For this review, take the finished solid that the model builds, in its own axes (mm). A direction names the side the tool comes from. Round coordinates to 2 decimals unless told otherwise and drop trailing zeros. Order: outer loops, then holes, each group sorted by start corner. A loop starts at its lowest first (then second) coordinate and runs counter-clockwise, first axis right, second up. Notation, with made-up numbers: (-33, -28.75) - (8, -28.75) arc R26 cw to (8, 4.25) - close; hole circle Ø2 at (50.25, 43). An arc over 180 degrees is marked (long way). One line per item, written item: value.
Autodesk Inventor part; units mm, degrees
ref_plane "YZ Plane" through (0, 0, 0) normal (1, 0, 0) x (0, 1, 0)
ref_plane "XZ Plane" through (0, 0, 0) normal (0, 1, 0) x (-1, 0, 0)
ref_plane "XY Plane" through (0, 0, 0) normal (0, 0, 1) x (1, 0, 0)
sketch "Esquisse3" plane through (0, 0, 0) normal (0, 1, 0) x (-1, 0, 0)
  line L0 (0, 0) -> (11.196, -1.161)
  line L1 (11.196, -1.161) -> (11.196, -3.161)
  line L2 (11.196, -3.161) -> (0, -2)
  line L3 (0, -2) -> (-8.226, -2.628)
  line L4 (-8.226, -2.628) -> (-8.226, -0.628)
  line L5 (-8.226, -0.628) -> (0, 0)
  line L6 (0, 0) -> (0, -2) construction
  dimension "d10" = 0.628
  dimension "d11" = 1.161
  dimension "d12" = 11.256
  dimension "d13" = 8.226
  dimension "d14" = 2
extrude "Extrusion1" add sketch "Esquisse3" along normal blind 8
ref_plane "Plan de construction1" through (0, 10, 0) normal (0, 1, 0) x (1, 0, 0)
sketch "Esquisse4" plane through (0, 10, 0) normal (0, 1, 0) x (1, 0, 0)
  line L0 (8.226, 0.628) -> (8.226, 2.628) construction
  line L1 (8.226, 2.628) -> (0, 2) construction
  line L2 (8.226, 2.628) -> (0, 2) construction
  line L3 (0, 2) -> (-11.196, 3.161) construction
  line L4 (0, 2) -> (-11.196, 3.161) construction
  line L5 (-11.196, 3.161) -> (-11.196, 4.661) construction
  line L6 (-11.196, 4.661) -> (0, 3.5)
  line L7 (0, 3.5) -> (8.226, 4.128)
  line L8 (8.226, 2.628) -> (8.226, 4.128) construction
  line L9 (0, 2) -> (0, 3.5) construction
  line L10 (-11.196, 4.661) -> (-11.196, 6.0463)
  line L11 (-11.196, 6.0463) -> (-0.0003, 4.8853)
  line L12 (-0.0003, 4.8853) -> (8.226, 5.5133)
  line L13 (8.226, 5.5133) -> (8.226, 4.128)
  point P0 (0, 0)
  dimension "d18" = 1.5
  dimension "d19" = 1.5
  dimension "d20" = 1.5
loft "Lissage1" add profiles "Esquisse4" section 1 edges at (-5.598, 8, -0.5805) (4.113, 8, -0.314) (8.226, 8, -1.628) (4.113, 8, -2.314) (-5.598, 8, -2.5805) (-11.196, 8, -2.161)
sketch "Esquisse9" plane through (0, 0, 0) normal (0, -1, 0) x (1, 0, 0)
  line L0 (8.226, -0.628) -> (0, 0)
  line L1 (8.226, -0.628) -> (0, 0)
  line L2 (0, 0) -> (-11.196, -1.161)
  line L3 (0, 0) -> (-11.196, -1.161)
  line L4 (-11.196, -1.161) -> (-11.196, -22.84)
  line L5 (-11.196, -22.84) -> (0, -24)
  line L6 (0, -24) -> (8.226, -23.371)
  line L7 (8.226, -0.628) -> (8.226, -2.628)
  line L8 (8.226, -23.371) -> (8.226, -0.628)
  line L9 (0, 0) -> (0, -24) construction
  dimension "d29" = 24
  dimension "d30" = 22.743
  dimension "d31" = 21.679
extrude "Extrusion2" add sketch "Esquisse9" against normal blind 1
sketch "Esquisse10" plane through (0, 0, 0) normal (0, -1, 0) x (1, 0, 0)
  line L0 (8.226, -15.371) -> (-11.774, -15.371)
  line L1 (-11.774, -15.371) -> (-11.774, -8.628)
  line L2 (-11.774, -8.628) -> (8.226, -8.628)
  line L3 (8.226, -8.628) -> (8.226, -15.371)
  point P0 (8.226, -23.371)
  point P1 (8.226, -0.628)
  dimension "d34" = 8
  dimension "d35" = 8
  dimension "d36" = 20
extrude "Extrusion3" add sketch "Esquisse10" against normal blind 1
ref_plane "Plan de construction3" through (-11.196, 0, -12.5995) normal (0, 0, -1) x (-1, 0, 0)
mirror "Symétrie2" about plane through (-11.196, 0, -12.5995) normal (0, 0, -1) of "Extrusion1", "Lissage1"
sketch "Esquisse11" plane through (0, 0, 0) normal (0, -1, 0) x (1, 0, 0)
  line L0 (8.226, -28.0995) -> (-1.774, -28.0995)
  line L1 (-1.774, -28.0995) -> (-1.774, 2.9005)
  line L2 (-1.774, 2.9005) -> (8.226, 2.9005)
  line L3 (8.226, 2.9005) -> (8.226, -28.0995) construction
  line L4 (8.226, -28.0995) -> (8.226, -24.571)
  line L5 (8.226, -24.571) -> (8.226, -0.628)
  line L6 (8.226, -0.628) -> (8.226, 2.9005)
  point P0 (0, 0)
  dimension "d40" = 31
  dimension "d41" = 10
extrude "Extrusion4" add sketch "Esquisse11" against normal blind 1
sketch "Esquisse12" plane through (0, 0, 0) normal (0, -1, 0) x (1, 0, 0)
  line L0 (8.226, -28.0995) -> (-1.774, -28.0995)
  line L1 (8.226, -28.0995) -> (-1.774, -28.0995)
  line L2 (-1.774, -28.0995) -> (-1.774, -26.0995)
  line L3 (-1.774, -28.0995) -> (-1.774, -25.015) construction
  line L4 (8.226, -24.571) -> (8.226, -28.0995) construction
  line L5 (8.226, -26.0995) -> (-1.774, -26.0995)
  line L6 (8.226, -28.0995) -> (8.226, -26.0995)
  point P0 (0, 0)
  dimension "d44" = 2
extrude "Extrusion5" add sketch "Esquisse12" along normal blind 8.5
mirror "Symétrie3" about plane through (-11.196, 0, -12.5995) normal (0, 0, -1) of "Extrusion5"
sketch "Esquisse13" plane through (0, -8.5, 0) normal (0, -1, 0) x (1, 0, 0)
  line L0 (8.226, -24.571) -> (8.226, -28.0995)
  line L1 (-1.774, 2.9005) -> (8.226, 2.9005)
  line L2 (8.226, -28.0995) -> (-1.774, -28.0995)
  line L3 (-1.774, -28.0995) -> (-1.774, 2.9005)
  line L4 (-1.774, 2.9005) -> (8.226, 2.9005)
  line L5 (8.226, 2.9005) -> (8.226, -28.0995)
  point P0 (0, 0)
extrude "Extrusion6" add sketch "Esquisse13" along normal blind 1
sketch "Esquisse14" plane through (0, -9.5, 0) normal (0, -1, 0) x (1, 0, 0)
  line L0 (-1.774, -26.0995) -> (-1.774, 0.9005) construction
  line L1 (8.226, 0.9005) -> (8.226, -26.0995) construction
  line L2 (-1.774, -20.0995) -> (8.226, -20.0995)
  line L3 (8.226, -20.0995) -> (8.226, -5.0995)
  line L4 (8.226, -5.0995) -> (-1.774, -5.0995)
  line L5 (-1.774, -5.0995) -> (-1.774, -20.0995)
  line L6 (-1.774, -28.0995) -> (8.226, -28.0995) construction
  line L7 (8.226, 2.9005) -> (-1.774, 2.9005) construction
  line L8 (-1.774, -20.0995) -> (-1.774, -5.0995)
  line L9 (8.226, -5.0995) -> (8.226, -20.0995)
  point P0 (0, 0)
  dimension "d49" = 8
  dimension "d50" = 8
extrude "Extrusion7" cut sketch "Esquisse14" against normal blind 1
properties part number "ESCFixation"
Item 1: Take a section at B-B (y = -7.5). Write out the cut boundary in (x, z).
Returned:
outline: (-1.77, -28.1) - (8.23, -28.1) - (8.23, -26.1) - (-1.77, -26.1) - close; (-1.77, 0.9) - (8.23, 0.9) - (8.23, 2.9) - (-1.77, 2.9) - close
Item 2: Machinability: for faces 5 (the flat face through (-5.68, 4.45, -2.59)), 6 (the flat face through (-11.196, 4, -3)), 7 (the flat face through (-1.6, 10, -4.6)), 8 (the flat face through (3, -8.5, -2)), 9 (the flat face through (3, -4, -28.1)), which of the approach directions +Z, -Z, +X, -X, +Y, -Y give a long, thin tool a straight path to every point of the face, cutting with its end or side? Answer none if there is none.
Returned:
face 5: none
face 6: +Z, -X, +Y, -Y
face 7: +Z, -Z, +X, -X, +Y
face 8: +X, -X
face 9: -Z, +X, -X, +Y, -Y
Item 3: For P1, Ø3, axis at x = -5.5, y = -1, coming from the +Z side; P2, Ø9, axis at y = -3, z = -24.5, coming from the -X side; P3, Ø1.8, axis at x = 2.5, z = 2, coming from the +Y side; P4, Ø1.5, axis at y = 2, z = -12, coming from the +X side, all flat-tipped, find the tip position at first contact; note any pin that passes through.
Returned:
P1: z = -0.45
P2: x = -11.2
P3: y = 1
P4: through
Item 4: Take a section at C-C (z = -9). Write out the cut boundary in (x, y).
Returned:
outline: (-11.77, 0) - (8.23, 0) - (8.23, 1) - (-11.77, 1) - close
Item 5: Take a section at A-A (y = 3). Write out the cut boundary in (x, z).
Returned:
outline: (-11.2, -24.04) - (0, -25.2) - (8.23, -24.57) - (8.23, -22.57) - (0, -23.2) - (-11.2, -22.04) - close; (-11.2, -3.16) - (0, -2) - (8.23, -2.63) - (8.23, -0.63) - (0, 0) - (-11.2, -1.16) - close
Item 6: The part is to be moulded in two halves that separate along X. For faces 1 (the flat face through (8.226, 0.3, -12.5)), 2 (the flat face through (-5.52, 4.451, -22.627)), 3 (the flat face through (3, -4, -26.1)), 4 (the flat face through (4.06, 4.45, -2.31)), say which applies: +X half, -X half, draft (parallel to the pull), parting line (faces both ways), or undercut.
Returned:
face 1: +X half
face 2: undercut
face 3: draft
face 4: undercut
Item 7: Wall thickness on line 1 (Y direction, x = 6.5, z = -21); line 2 (Y direction, x = 7.75, z = -26); line 3 (Z direction, x = -0.25, y = -0.5): over which ranges is each line inside the solid? List them lowest first.
Returned:
line 1: -9.5 to -8.5, 0 to 1, 9.18 to 10
line 2: -9.5 to -8.5, 0 to 1
line 3: -28.1 to -26.1, 0.9 to 2.9
